Design review of the part built by this model. Coordinates are the model's own, in mm. A direction names the side the tool comes from. Coordinates: 2 decimals unless noted, no trailing zeros. Loops run counter-clockwise (first coordinate to the right, second up) from the corner with the lowest first, then second, coordinate; pieces in that order, holes last. Notation, with made-up numbers: (17, 54.5) -> (50, 54.5) arc R20 ccw to (50, 65.5) -> close; hole circle Ø1 at (-22, 36). An arc over 180 degrees is marked (long way). One line per item, written item: value. Start each with the question number.
1. Add section A-A on y = 0. Write out the cut boundary in (x, z).
2. Insertion check: pin 1 (1.5 mm diameter, centred on x = 2, z = 3.5, fed in from -Y) (3 decimals); pin 2 (8 mm diameter, centred on y = -4.5, z = 4, fed in from +X); pin 3 (4 mm diameter, centred on x = -8, z = 9.5, fed in from +Y); pin 4 (8 mm diameter, centred on y = -4, z = 1, fed in from -X). Each pin has a flat end and moves straight along its axis. Give the tip position at first contact, or say it passes through.
3. For probe 1 along Y at (x, z) = (0, 8.25); probe 2 along Y at (x, z) = (0, 0.75); probe 3 along Z at (x, y) = (10, -3), list the stretches that pass through material, from the lowest coordinate up.
4. Draft analysis for pull direction Y (two halves, no side actions). For faces 4 (the cylindrical face through (-6, 0, -2)), 5 (the flat face through (5, 0, 13)), 6 (the cylindrical face through (-0.59, 4.46, 4.13)), state which applies: pulls with the +Y half, pulls with the -Y half, needs draft (parallel to the pull), parting line crosses it, or undercut.
5. Add section C-C on z = 4.5. Write out the cut boundary in (x, y), plus the area to 3 significant figures.
6. Machinability: for faces 1 (the flat face through (7, 0, 0)), 2 (the cylindrical face through (-3.47, -15.62, 1.48)), 3 (the cylindrical face through (10, 3.2, 7.9)), which of the approach directions +Z, -Z, +X, -X, +Y, -Y give a long, thin tool a straight path to every point of the face, cutting with its end or side? Answer none if there is none.
7. Add section D-D on y = -5.5. Write out the cut boundary in (x, z), plus the area to 3 significant figures.
```python
from build123d import *

# Parameters (mm, degrees)
SKETCH_R     = 16
PAD_DEPTH    = 3
SKETCH001_R  = 10.5
PAD001_DEPTH = 10
SKETCH002_R  = 6
PAD002_DEPTH = 5
SKETCH003_R  = 4.5
POCKET_DEPTH = 18.001


with BuildPart() as part:
    # Sketch → Pad (new body)
    with BuildSketch(Plane.XY):
        Circle(SKETCH_R)
    extrude(amount=PAD_DEPTH)

    # Sketch001 (on Face3 of Pad) → Pad001 (join)
    with BuildSketch(Plane.XY.offset(3)):
        Circle(SKETCH001_R)
    extrude(amount=PAD001_DEPTH)

    # Sketch002 (on Face2 of Pad001) → Pad002 (join)
    with BuildSketch(Plane(origin=(0, 0, 0), x_dir=(1, 0, 0), z_dir=(0, 0, -1))):
        Circle(SKETCH002_R)
    extrude(amount=PAD002_DEPTH)

    # Sketch003 (on Face7 of Pad002) → Pocket (cut, through all)
    with BuildSketch(Plane.XY.offset(13)):
        Circle(SKETCH003_R)
    extrude(amount=-POCKET_DEPTH, mode=Mode.SUBTRACT)


solid = part.part
```
Worked answers:
1. outline: (-16, 0) -> (-6, 0) -> (-6, -5) -> (-4.5, -5) -> (-4.5, 13) -> (-10.5, 13) -> (-10.5, 3) -> (-16, 3) -> close; (4.5, -5) -> (6, -5) -> (6, 0) -> (16, 0) -> (16, 3) -> (10.5, 3) -> (10.5, 13) -> (4.5, 13) -> close
2. pin 1: stops at y = -15.935
2. pin 2: stops at x = 15.99
2. pin 3: stops at y = 8.62
2. pin 4: stops at x = -16
3. probe 1: y = -10.5 to -4.5, 4.5 to 10.5
3. probe 2: y = -16 to -4.5, 4.5 to 16
3. probe 3: z = 0 to 13
4. face 4: parting line crosses it
4. face 5: needs draft
4. face 6: undercut
5. outline: circle Ø21 at (0, 0); hole circle Ø9 at (0, 0)
5. area: 283 mm²
6. face 1: -Z
6. face 2: +Z, -Z
6. face 3: +Z
7. outline: (-15.02, 0) -> (-2.4, 0) -> (-2.4, -5) -> (2.4, -5) -> (2.4, 0) -> (15.02, 0) -> (15.02, 3) -> (8.94, 3) -> (8.94, 13) -> (-8.94, 13) -> (-8.94, 3) -> (-15.02, 3) -> close
7. area: 293 mm²
